from build123d import *

# Parameters (mm, degrees)
BOSS_EXTRUDE1_DEPTH = 5
SKETCH4_R           = 6.430810597
CUT_EXTRUDE2_DEPTH  = 10
SKETCH2_W           = 20
SKETCH2_H           = 9.116342764
BOSS_EXTRUDE2_DEPTH = 10
SKETCH3_R           = 3
CUT_EXTRUDE1_DEPTH  = 49.586866564
CIRPATTERN1_COUNT   = 3


with BuildPart() as part:
    # Sketch1 → Boss-Extrude1 (new body)
    with BuildSketch(Plane(origin=(0, 0, 0), x_dir=(1, 0, 0), z_dir=(0, 1, 0))):
        Polygon((14.43375673, 25), (-14.43375673, 25), (-28.867513459, 0), (-14.43375673, -25), (14.43375673, -25), (28.867513459, 0), align=None)
    extrude(amount=BOSS_EXTRUDE1_DEPTH)

    # Sketch4 → Cut-Extrude2 (cut)
    with BuildSketch(Plane(origin=(0, 5, 0), x_dir=(1, 0, 0), z_dir=(0, 1, 0))):
        with Locations(Location((0, 0, 0), (0, 0, 270))):
            Circle(SKETCH4_R)
    extrude(amount=-CUT_EXTRUDE2_DEPTH, mode=Mode.SUBTRACT)

    # Sketch2 → Boss-Extrude2 (add)
    with BuildSketch(Plane(origin=(0, 5, 0), x_dir=(1, 0, 0), z_dir=(0, 1, 0))):
        with Locations((0, -20.441828618)):
            Rectangle(SKETCH2_W, SKETCH2_H)
    boss_extrude2 = extrude(amount=BOSS_EXTRUDE2_DEPTH)

    # Sketch3 → Cut-Extrude1 (cut, through all)
    with BuildSketch(Plane(origin=(10, 0, 0), x_dir=(0, 0, -1), z_dir=(1, 0, 0))):
        with Locations((-20.441828618, 10)):
            Circle(SKETCH3_R)
    cut_extrude1 = extrude(amount=-CUT_EXTRUDE1_DEPTH, mode=Mode.SUBTRACT)

    # CirPattern1: Boss-Extrude2, Cut-Extrude1 ×3 about axis
    cirpattern1_axis = Axis((0, 0, 0), (0, 1, 0))
    add([boss_extrude2.rotate(cirpattern1_axis, i * 360 / CIRPATTERN1_COUNT) for i in range(1, CIRPATTERN1_COUNT)])
    add([cut_extrude1.rotate(cirpattern1_axis, i * 360 / CIRPATTERN1_COUNT) for i in range(1, CIRPATTERN1_COUNT)], mode=Mode.SUBTRACT)


solid = part.part
Work out the finished part from the listing and answer in its coordinate system (mm). A direction names the side the tool comes from. Round coordinates to 2 decimals unless told otherwise and drop trailing zeros. Write each loop counter-clockwise with the first axis right and the second up, starting at its lowest first coordinate (ties: lowest second). Pieces come first, ordered by that corner, then holes. Notation, with made-up numbers: (70, -14.5) -> (125, -14.5) arc R32 cw to (125, 15.5) -> close; hole circle Ø7 at (60.5, 86.5). An arc over 180 degrees is marked (long way). Answer as CSV lines item,"result". Start each with the question number.
(1) The mould has two halves that part along Z. Classify faces 6 (the flat face through (25.39, 8.82, -3.11)), 7 (the cylindrical face through (0.14, 10.13, 23.44)), 8 (the flat face through (0, 2, -25)): +Z half, -Z half, draft (parallel to the pull), parting line (faces both ways), or undercut.
(2) Find the intervals of material crossed by probe 1 along X at (y, z) = (3.15, 0); probe 2 along X at (y, z) = (9.25, -11); probe 3 along Z at (x, y) = (-0.5, 1.75), in increasing order.
(3) The part is cut by section B-B, the plane x = 0. Give the vertices of the cut face in (y, z).
(4) A tool of negligible diameter and unlimited length cuts with its end or side. For faces 1 (the flat face through (-25.39, 8.82, -3.11)), 2 (the flat face through (15.39, 8.819, -20.432)), 3 (the flat face through (-7, 5, 0)), 4 (the flat face through (6, 0, -6)), 5 (the flat face through (10, 8, 23)), from which of +Z, -Z, +X, -X, +Y, -Y can it reach the whole face along a straight path? Write none if from no direction.
(5) The part is cut by section D-D, the plane y = 8.25. Give the vertices of the cut face in (x, z).
(6) The part is cut by section C-C, the plane y = 14.25. Give the vertices of the cut face in (x, z), then the cut area to 3 significant figures.
(7) The part is cut by section A-A, the plane y = 2. Give the vertices of the cut face in (x, z).
(8) Each of these flat-tipped pins is pushed along its axis until it touches: pin 1 (8 mm diameter, centred on x = -5, y = 11, fed in from -Z); pin 2 (7.5 mm diameter, centred on y = 11, z = 20, fed in from +X); pin 3 (1 mm diameter, centred on x = -16.5, y = 1.5, fed in from -Z). Where does it stop, or does it pass through?
Output values:
1,face 6,"+Z half"
1,face 7,"undercut"
1,face 8,"-Z half"
2,probe 1,"x = -28.87 to -6.43, 6.43 to 28.87"
2,probe 2,"x = -22.52 to -20.61, -13.9 to -11.99, 11.99 to 13.9, 20.61 to 22.52"
2,probe 3,"z = -25 to -6.41, 6.41 to 25"
3,outline,"(0, -25) -> (5, -25) -> (5, -6.43) -> (0, -6.43) -> close; (0, 6.43) -> (5, 6.43) -> (5, 15.88) -> (15, 15.88) -> (15, 25) -> (0, 25) -> close; hole circle Ø6 at (10, 20.44)"
4,face 1,"+Z, -X, +Y"
4,face 2,"-Z, +Y"
4,face 3,"+Y"
4,face 4,"+Z, -Z, +X, -X, -Y"
4,face 5,"+Z, +X, +Y"
5,outline,"(-26.65, -3.84) -> (-16.65, -21.16) -> (-14.81, -20.1) -> (-24.81, -2.78) -> close; (-20.59, -0.34) -> (-10.59, -17.66) -> (-8.76, -16.6) -> (-18.76, 0.72) -> close; (-10, 15.88) -> (10, 15.88) -> (10, 18.01) -> (-10, 18.01) -> close; (-10, 22.88) -> (10, 22.88) -> (10, 25) -> (-10, 25) -> close; (8.76, -16.6) -> (10.59, -17.66) -> (20.59, -0.34) -> (18.76, 0.72) -> close; (14.81, -20.1) -> (16.65, -21.16) -> (26.65, -3.84) -> (24.81, -2.78) -> close"
6,outline,"(-26.65, -3.84) -> (-16.65, -21.16) -> (-8.76, -16.6) -> (-18.76, 0.72) -> close; (-10, 15.88) -> (10, 15.88) -> (10, 25) -> (-10, 25) -> close; (8.76, -16.6) -> (16.65, -21.16) -> (26.65, -3.84) -> (18.76, 0.72) -> close"
6,area,"547 mm²"
7,outline,"(-28.87, 0) -> (-14.43, -25) -> (14.43, -25) -> (28.87, 0) -> (14.43, 25) -> (-14.43, 25) -> close; hole circle Ø12.86 at (0, 0)"
8,pin 1,"stops at z = -16.74"
8,pin 2,"stops at x = 10"
8,pin 3,"stops at z = -22.29"
